```python
from build123d import *

# Parameters (mm, degrees)
BOSS_EXTRUDE1_DEPTH = 7
SKETCH3_R           = 2.7
CUT_EXTRUDE1_DEPTH  = 47.626172907
SKETCH4_R           = 2.7
CUT_EXTRUDE2_DEPTH  = 47.626172907


with BuildPart() as part:
    # Sketch1 → Boss-Extrude1 (new, symmetric)
    with BuildSketch(Plane.XY):
        with BuildLine():
            Line((0, 35), (0, 0))
            Line((0, 0), (35, 0))
            Line((35, 0), (35, 5))
            Line((35, 5), (15.8, 5))
            Line((15.8, 5), (12.2, 8.6))
            ThreePointArc((12.2, 8.6), (14.596011157, 10.003433414), (15.072479467, 12.739027089))
            Line((15.072479467, 12.739027089), (13.913368476, 12.428444235))
            ThreePointArc((13.913368476, 12.428444235), (10.4, 10.4), (12.428444235, 13.913368476))
            Line((12.428444235, 13.913368476), (12.739027089, 15.072479467))
            ThreePointArc((12.739027089, 15.072479467), (10.003433414, 14.596011157), (8.6, 12.2))
            Line((8.6, 12.2), (5, 15.8))
            Line((5, 15.8), (5, 35))
            Line((5, 35), (0, 35))
        make_face()
    extrude(amount=BOSS_EXTRUDE1_DEPTH, both=True)

    # Sketch3 → Cut-Extrude1 (cut, through all)
    with BuildSketch(Plane(origin=(0, 5, 0), x_dir=(1, 0, 0), z_dir=(0, 1, 0))):
        with Locations(Location((26, 0, 0), (0, 0, 180))):
            Circle(SKETCH3_R)
    extrude(amount=-CUT_EXTRUDE1_DEPTH, mode=Mode.SUBTRACT)

    # Sketch4 → Cut-Extrude2 (cut, through all)
    with BuildSketch(Plane(origin=(5, 0, 0), x_dir=(0, 0, -1), z_dir=(1, 0, 0))):
        with Locations((0, 26)):
            Circle(SKETCH4_R)
    extrude(amount=-CUT_EXTRUDE2_DEPTH, mode=Mode.SUBTRACT)


solid = part.part
```
Design review of the part built by this model. Coordinates are the model's own, in mm. A direction names the side the tool comes from. Coordinates: 2 decimals unless noted, no trailing zeros. Order: outer loops, then holes, each group sorted by start corner. A loop starts at its lowest first (then second) coordinate and runs counter-clockwise, first axis right, second up. Notation, with made-up numbers: (-20, -0.75) - (-8, -0.75) arc R26 ccw to (-8, 36.25) - close; hole circle Ø10 at (25, 78). An arc over 180 degrees is marked (long way). Answer in a Markdown table with one row per item.
(1) Wall thickness on line 1 along Y through (x, z) = (12, 3); line 2 along X through (y, z) = (16, -4.25); line 3 along Y through (x, z) = (3.3, 0): over which ranges is each line inside the solid? List them lowest first. Write a range as from..to.
Checked values:
| item | result |
|---|---|
| line 1 | 0..9.79, 13.98..15.18 |
| line 2 | 0..5 |
| line 3 | 0..23.3, 28.7..35 |
(2) Consider section C-C on z = 0. State the section outline as (x, y) points, plus the area to 3 significant figures.
Checked values:
| item | result |
|---|---|
| outline | (0, 0) - (23.3, 0) - (23.3, 5) - (15.8, 5) - (12.2, 8.6) arc R3.3 ccw to (15.07, 12.74) - (13.91, 12.43) arc R2.1 cw (long way) to (12.43, 13.91) - (12.74, 15.07) arc R3.3 ccw to (8.6, 12.2) - (5, 15.8) - (5, 23.3) - (0, 23.3) - close; (0, 28.7) - (5, 28.7) - (5, 35) - (0, 35) - close; (28.7, 0) - (35, 0) - (35, 5) - (28.7, 5) - close |
| area | 342 mm^2 |
(3) For faces 4 (the flat face through (14, 6.8, 0.1)), 5 (the flat face through (6.8, 14, 0.1)), 6 (the flat face through (23, 5, 2)), list the 3-axis set-ups (+Z, -Z, +X, -X, +Y, -Y) from which the entire face can be reached by the end or side of a thin tool; tool diameter is ignored.
Checked values:
| item | result |
|---|---|
| face 4 | +Z, -Z, +X |
| face 5 | +Z, -Z, +Y |
| face 6 | +Z, -Z, +X, +Y |
(4) The part is to be moulded in two halves that separate along Y. For faces 1 (the flat face through (11, 9, 7)), 2 (the cylindrical face through (2.535, 28.677, 0.351)), 3 (the flat face through (17, 0, 0)), say which applies: released by +Y, released by -Y, zero draft, split by the parting line, or undercut.
Checked values:
| item | result |
|---|---|
| face 1 | zero draft |
| face 2 | undercut |
| face 3 | released by -Y |
(5) Consider section A-A on x = 26. State the section outline as (y, z) points, plus the area to 3 significant figures.
Checked values:
| item | result |
|---|---|
| outline | (0, -7) - (5, -7) - (5, -2.7) - (0, -2.7) - close; (0, 2.7) - (5, 2.7) - (5, 7) - (0, 7) - close |
| area | 43.0 mm^2 |
(6) Consider section D-D on z = -5.25. State the section outline as (x, y) points.
Checked values:
| item | result |
|---|---|
| outline | (0, 0) - (35, 0) - (35, 5) - (15.8, 5) - (12.2, 8.6) arc R3.3 ccw to (15.07, 12.74) - (13.91, 12.43) arc R2.1 cw (long way) to (12.43, 13.91) - (12.74, 15.07) arc R3.3 ccw to (8.6, 12.2) - (5, 15.8) - (5, 35) - (0, 35) - close |
(7) Clearance check with flat-ended pins moving along their axes: pin 1 (4 mm diameter, centred on x = 25, z = -1.5, fed in from +Y); pin 2 (3 mm diameter, centred on y = 5.5, z = 1.5, fed in from +X); pin 3 (4 mm diameter, centred on y = 29.5, z = -1.5, fed in from +X); pin 4 (2 mm diameter, centred on x = 13, z = 4, fed in from +Y). State where each tip first meets the part, or that it passes through.
Checked values:
| item | result |
|---|---|
| pin 1 | y = 5 |
| pin 2 | x = 35 |
| pin 3 | x = 5 |
| pin 4 | y = 15.18 |
